from build123d import *

# Parameters (mm, degrees)
F1_DEPTH = 200
F2_R     = 8.5
F3_DEPTH = 10.001
F4_W     = 70
F4_H     = 10
F5_DEPTH = 70
F7_DEPTH = 10
F8_R     = 2


with BuildPart() as f1:
    # F0 (on Top) → F1 (new body)
    with BuildSketch(Plane.XY):
        Polygon((-12.944079712, 104.5888163149), (-22.944079712, 104.5888163149), (-22.944079712, -95.4111836851), (-12.944079712, -95.4111836851), (-12.944079712, 17.7888163149), (97.055920288, 17.7888163149), (97.055920288, 27.7888163149), (-12.944079712, 27.7888163149), align=None)
    extrude(amount=F1_DEPTH)

    # F2 (on face) → F3 (cut, through all)
    with BuildSketch(Plane.YZ.offset(-12.944079712)):
        with Locations((89.5888163149, 185)):
            Circle(F2_R)
        with Locations((89.5888163149, 15)):
            Circle(F2_R)
        with Locations((-80.4111836851, 15)):
            Circle(F2_R)
        with Locations((-80.4111836851, 185)):
            Circle(F2_R)
    extrude(amount=-F3_DEPTH, mode=Mode.SUBTRACT)

    # F4 (on face) → F5 (join)
    with BuildSketch(Plane.YZ.offset(-12.944079712)):
        with Locations((-17.2111836851, 100)):
            Rectangle(F4_W, F4_H)
    extrude(amount=F5_DEPTH)

    # F6 (on face) → F7 (cut)
    with BuildSketch(Plane.XY.offset(105)):
        Polygon((57.055920288, 17.7888163149), (-12.944079712, -52.2111836851), (57.055920288, -52.2111836851), align=None)
    extrude(amount=-F7_DEPTH, mode=Mode.SUBTRACT)

    # F8
    f8_edges = [f1.edges().sort_by_distance(p)[0] for p in [
        (-12.94408, 17.788816, 152.5),
        (-12.94408, -17.211184, 105),
        (-12.94408, -17.211184, 95),
        (-12.94408, 17.788816, 47.5),
        (-12.94408, 27.788816, 100),
        (57.05592, 17.788816, 100),
        (22.05592, 17.788816, 105),
        (22.05592, 17.788816, 95),
    ]]
    fillet(f8_edges, radius=F8_R)


solid = f1.part
Geometry check sheet. Reference: the model listing, model coordinates, mm. A direction names the side the tool comes from. Round coordinates to 2 decimals unless told otherwise and drop trailing zeros. Loops run counter-clockwise (first coordinate to the right, second up) from the corner with the lowest first, then second, coordinate; pieces in that order, holes last. Notation, with made-up numbers: (40.25, 59) -> (77.25, 59) arc R12 ccw to (77.25, 74) -> close; hole circle Ø6 at (11.25, 15.25). An arc over 180 degrees is marked (long way). Answer as a JSON object with one key per item and string values. Group by question number.
Item 1: Cross-section at D-D, the plane y = -19.5. Record the cut outline in (x, z), plus the area to 3 significant figures.
Item 2: Thickness scan on line 1 along Y through (x, z) = (-15.5, 11); line 2 along Z through (x, y) = (-17, -78.5); line 3 along Y through (x, z) = (24.5, 126.5). Record the ranges inside material, lowest first.
Item 3: Cross-section at B-B, the plane z = 99.5. Record the cut outline in (x, y), plus the area to 3 significant figures.
Item 4: Cross-section at C-C, the plane x = 51. Record the cut outline in (y, z), plus the area to 3 significant figures.
Item 5: Set-up check for faces 1 (the face through (10, 20, 0)), 2 (the face through (44, 27.789, 99)), 3 (the face through (7, -3, 105)), 4 (the face through (42, 17.789, 76)): record each of +Z, -Z, +X, -X, +Y, -Y from which the full face is reachable in a straight line by a thin tool's end or side.
Item 6: Release check for a two-part mould opening along Z. For faces 5 (the face through (7, -3, 95)), 6 (the face through (-12.944, 67, 99)), 7 (the face through (-17.87, -82.25, 176.7)) record: pulls with the +Z half, pulls with the -Z half, needs draft (parallel to the pull), parting line crosses it, or undercut.
Item 7: Depth check by flat-ended pin: pin 1 Ø1.5 at (x, z) = (67.5, 84.5) entering from -Y; pin 2 Ø10 at (y, z) = (-80.41, 15) entering from +X; pin 3 Ø3 at (y, z) = (-63.5, 135) entering from +X. Enter the tip coordinate at first touch or a pass-through.
Item 8: Cross-section at A-A, the plane z = 15. Record the cut outline in (x, y), plus the area to 3 significant figures.
Determined:
{
 "1": {"outline": "(-22.94, 0) -> (-12.94, 0) -> (-12.94, 93) arc R2 cw to (-10.94, 95) -> (19.77, 95) -> (19.77, 105) -> (-10.94, 105) arc R2 cw to (-12.94, 107) -> (-12.94, 200) -> (-22.94, 200) -> close", "area": "2,330 mm²"},
 "2": {"line 1": "y = -95.41 to -87.91, -72.91 to 82.09, 97.09 to 104.59", "line 2": "z = 0 to 6.72, 23.28 to 176.72, 193.28 to 200", "line 3": "y = 17.79 to 27.79"},
 "3": {"outline": "(-22.94, -95.41) -> (-12.94, -95.41) -> (-12.94, -52.21) -> (56.47, 17.2) arc R2 cw to (57.88, 17.79) -> (97.06, 17.79) -> (97.06, 27.79) -> (-10.94, 27.79) arc R2 cw to (-12.94, 29.79) -> (-12.94, 104.59) -> (-22.94, 104.59) -> close", "area": "5,550 mm²"},
 "4": {"outline": "(11.73, 95) -> (15.79, 95) arc R2 cw to (17.79, 93) -> (17.79, 0) -> (27.79, 0) -> (27.79, 200) -> (17.79, 200) -> (17.79, 107) arc R2 cw to (15.79, 105) -> (11.73, 105) -> close", "area": "2,060 mm²"},
 "5": {"face 1": "-Z, +X, -X, +Y, -Y", "face 2": "+Z, -Z, +X, +Y", "face 3": "+Z, +X, -Y", "face 4": "+X, -Y"},
 "6": {"face 5": "pulls with the -Z half", "face 6": "needs draft", "face 7": "undercut"},
 "7": {"pin 1": "stops at y = 17.79", "pin 2": "passes through", "pin 3": "stops at x = -12.94"},
 "8": {"outline": "(-22.94, -95.41) -> (-12.94, -95.41) -> (-12.94, -88.91) -> (-22.94, -88.91) -> close; (-22.94, -71.91) -> (-12.94, -71.91) -> (-12.94, 15.79) arc R2 cw to (-10.94, 17.79) -> (97.06, 17.79) -> (97.06, 27.79) -> (-10.94, 27.79) arc R2 cw to (-12.94, 29.79) -> (-12.94, 81.09) -> (-22.94, 81.09) -> close; (-22.94, 98.09) -> (-12.94, 98.09) -> (-12.94, 104.59) -> (-22.94, 104.59) -> close", "area": "2,760 mm²"}
}
